from build123d import *

# Parameters (mm, degrees)
F0_W     = 16.8741471134
F0_H     = 2.6543606073
F0_W_2   = 2.2751651704
F0_H_2   = 12.3238116503
F0_W_3   = 16.8741438538
F0_H_3   = 3.0335541815
F0_W_4   = 2.6543606073
F0_H_4   = 3.9815418422
F0_H_5   = 11.5654245019
F0_W_5   = 11.7550231516
F0_W_6   = 7.0150978863
F0_H_6   = 1.8959715962
F0_W_7   = 2.2786548152
F0_H_7   = 3.3179512247
F0_H_8   = 7.4890879914
F0_W_8   = 11.5619385824
F0_W_9   = 2.8439611197
F0_H_9   = 7.7734831721
F0_H_10  = 2.9387557879
F0_H_11  = 8.0578802153
F0_W_10  = 11.3758221269
F1_DEPTH = 7.62
F2_DEPTH = 8.382
F4_DEPTH = 25.4


with BuildPart() as f1:
    # F0 (on Front) → F1 (new body)
    with BuildSketch(Plane.XZ):
        Polygon((-41.2373803556, 39.1518138349), (-41.2373803556, 41.4269790053), (-46.7357002199, 41.4269790053), (-52.4236150086, 39.5310074091), (-54.8883751035, 35.1702719927), (-54.8883751035, 26.8279965967), (-54.8883751035, 18.2961262763), (-50.5276434124, 15.2625711635), (-46.1669079959, 15.2625711635), (-41.9957712293, 15.2625711635), (-35.9286628664, 15.2625711635), (-30.6199416518, 15.0729743764), (-35.7390642166, 18.2961262763), (-41.2373803556, 18.2961262763), (-49.5796576142, 18.2961262763), (-52.4236150086, 20.3816946596), (-52.4236150086, 25.8800126612), (-52.4236150086, 34.0326912701), (-50.7172383368, 36.8766486645), (-45.2189221978, 39.1518138349), align=None)
        Polygon((-35.7390642166, 34.7910784185), (-35.7390642166, 18.2961262763), (-30.6199416518, 15.0729743764), (-20.9504868835, 15.0729743764), (-17.5377372652, 18.2961262763), (-15.4521688819, 21.7088758945), (-15.4521688819, 32.5159132481), (-15.4521688819, 38.2038280368), (-17.5377372652, 41.6165776551), (-23.415248841, 41.6165776551), (-27.3967888206, 41.4269790053), (-31.9471210241, 41.4269790053), (-35.1702719927, 38.3934266865), align=None)
        Polygon((-17.5377372652, 18.2961262763), (-20.9504868835, 15.0729743764), (-10.1434476674, 15.0729743764), (-10.1434476674, 17.5377372652), align=None)
        Polygon((-10.1434476674, 17.5377372652), (-10.1434476674, 15.0729743764), (-7.6786852442, 14.883376658), (-7.6786852442, 17.5377372652), (-7.6786852442, 36.3078564405), (-10.1434476674, 36.3078564405), align=None)
        with Locations((0.7583883125, 16.2105569616)):
            Rectangle(F0_W, F0_H)
        Polygon((-10.1434476674, 40.2893982828), (-10.1434476674, 36.3078564405), (-7.6786852442, 36.3078564405), (2.3699654266, 36.3078564405), (2.3699654266, 40.2893982828), (-7.8682824969, 40.2893982828), align=None)
        Polygon((9.1954618692, 17.5377372652), (9.1954618692, 14.883376658), (11.8498224765, 14.6937798709), (11.8498224765, 17.7273340523), (11.8498224765, 36.6870500147), (9.1954618692, 36.6870500147), align=None)
        with Locations((-9.0058650821, 46.4513041079)):
            Rectangle(F0_W_2, F0_H_2)
        with Locations((20.2868944034, 16.2105569616)):
            Rectangle(F0_W_3, F0_H_3)
        Polygon((-10.1434476674, 56.0259595513), (-10.1434476674, 52.613209933), (-7.8682824969, 52.613209933), (6.9202957675, 52.613209933), (6.9202957675, 56.0259595513), align=None)
        with Locations((10.5226421729, 38.6778209358)):
            Rectangle(F0_W_4, F0_H_4)
        Polygon((28.7239663303, 17.7273340523), (28.7239663303, 14.6937798709), (42.5645597279, 14.6937798709), (42.5645597279, 16.5897514671), (42.5645597279, 18.1065294892), (31.0026211455, 17.789763132), align=None)
        with Locations((10.5226421729, 46.4513041079)):
            Rectangle(F0_W_4, F0_H_5)
        with Locations((17.7273340523, 38.6778209358)):
            Rectangle(F0_W_5, F0_H_4)
        Polygon((28.7239663303, 25.5008172244), (28.7239663303, 17.7273340523), (31.0026211455, 17.789763132), (31.0026211455, 25.5008172244), align=None)
        with Locations((46.0721086711, 15.641765669)):
            Rectangle(F0_W_6, F0_H_6)
        Polygon((9.1954618692, 56.0259595513), (9.1954618692, 52.2340163589), (11.8498224765, 52.2340163589), (26.2592080981, 52.2340163589), (26.2592080981, 56.0259595513), align=None)
        with Locations((29.8632937379, 27.1597928368)):
            Rectangle(F0_W_7, F0_H_7)
        Polygon((49.5796576142, 16.5897514671), (49.5796576142, 14.6937798709), (63.6098459363, 14.6937798709), (63.6098459363, 18.1065294892), (52.4236187339, 18.1065294892), (49.5796576142, 18.1065294892), align=None)
        with Locations((29.8632937379, 32.5633124448)):
            Rectangle(F0_W_7, F0_H_8)
        with Locations((36.7835904367, 27.1597928368)):
            Rectangle(F0_W_8, F0_H_7)
        Polygon((28.7239663303, 39.9102028459), (28.7239663303, 36.3078564405), (31.0026211455, 36.3078564405), (42.5645597279, 36.3078564405), (42.5645597279, 39.9102028459), align=None)
        with Locations((51.0016381741, 21.9932710752)):
            Rectangle(F0_W_9, F0_H_9)
        with Locations((51.0016381741, 27.3493905552)):
            Rectangle(F0_W_9, F0_H_10)
        with Locations((51.0016381741, 32.8477085568)):
            Rectangle(F0_W_9, F0_H_11)
        with Locations((58.1115297973, 27.3493905552)):
            Rectangle(F0_W_10, F0_H_10)
        Polygon((49.5796576142, 39.9102047086), (49.5796576142, 36.8766486645), (52.4236187339, 36.8766486645), (63.9890432358, 36.8766486645), (63.9890432358, 39.9102047086), align=None)
    extrude(amount=F1_DEPTH)

    # F0 (on Front) → F2 (join)
    with BuildSketch(Plane.XZ):
        Polygon((-41.2373803556, 39.1518138349), (-41.2373803556, 41.4269790053), (-46.7357002199, 41.4269790053), (-52.4236150086, 39.5310074091), (-54.8883751035, 35.1702719927), (-54.8883751035, 26.8279965967), (-54.8883751035, 18.2961262763), (-50.5276434124, 15.2625711635), (-46.1669079959, 15.2625711635), (-41.9957712293, 15.2625711635), (-35.9286628664, 15.2625711635), (-30.6199416518, 15.0729743764), (-35.7390642166, 18.2961262763), (-41.2373803556, 18.2961262763), (-49.5796576142, 18.2961262763), (-52.4236150086, 20.3816946596), (-52.4236150086, 25.8800126612), (-52.4236150086, 34.0326912701), (-50.7172383368, 36.8766486645), (-45.2189221978, 39.1518138349), align=None)
        Polygon((-35.7390642166, 34.7910784185), (-35.7390642166, 18.2961262763), (-30.6199416518, 15.0729743764), (-20.9504868835, 15.0729743764), (-17.5377372652, 18.2961262763), (-15.4521688819, 21.7088758945), (-15.4521688819, 32.5159132481), (-15.4521688819, 38.2038280368), (-17.5377372652, 41.6165776551), (-23.415248841, 41.6165776551), (-27.3967888206, 41.4269790053), (-31.9471210241, 41.4269790053), (-35.1702719927, 38.3934266865), align=None)
        Polygon((-17.5377372652, 18.2961262763), (-20.9504868835, 15.0729743764), (-10.1434476674, 15.0729743764), (-10.1434476674, 17.5377372652), align=None)
        Polygon((-10.1434476674, 17.5377372652), (-10.1434476674, 15.0729743764), (-7.6786852442, 14.883376658), (-7.6786852442, 17.5377372652), (-7.6786852442, 36.3078564405), (-10.1434476674, 36.3078564405), align=None)
        with Locations((0.7583883125, 16.2105569616)):
            Rectangle(F0_W, F0_H)
        Polygon((-10.1434476674, 40.2893982828), (-10.1434476674, 36.3078564405), (-7.6786852442, 36.3078564405), (2.3699654266, 36.3078564405), (2.3699654266, 40.2893982828), (-7.8682824969, 40.2893982828), align=None)
        Polygon((9.1954618692, 17.5377372652), (9.1954618692, 14.883376658), (11.8498224765, 14.6937798709), (11.8498224765, 17.7273340523), (11.8498224765, 36.6870500147), (9.1954618692, 36.6870500147), align=None)
        with Locations((-9.0058650821, 46.4513041079)):
            Rectangle(F0_W_2, F0_H_2)
        with Locations((20.2868944034, 16.2105569616)):
            Rectangle(F0_W_3, F0_H_3)
        Polygon((-10.1434476674, 56.0259595513), (-10.1434476674, 52.613209933), (-7.8682824969, 52.613209933), (6.9202957675, 52.613209933), (6.9202957675, 56.0259595513), align=None)
        with Locations((10.5226421729, 38.6778209358)):
            Rectangle(F0_W_4, F0_H_4)
        Polygon((28.7239663303, 17.7273340523), (28.7239663303, 14.6937798709), (42.5645597279, 14.6937798709), (42.5645597279, 16.5897514671), (42.5645597279, 18.1065294892), (31.0026211455, 17.789763132), align=None)
        with Locations((10.5226421729, 46.4513041079)):
            Rectangle(F0_W_4, F0_H_5)
        with Locations((17.7273340523, 38.6778209358)):
            Rectangle(F0_W_5, F0_H_4)
        Polygon((28.7239663303, 25.5008172244), (28.7239663303, 17.7273340523), (31.0026211455, 17.789763132), (31.0026211455, 25.5008172244), align=None)
        with Locations((46.0721086711, 15.641765669)):
            Rectangle(F0_W_6, F0_H_6)
        Polygon((9.1954618692, 56.0259595513), (9.1954618692, 52.2340163589), (11.8498224765, 52.2340163589), (26.2592080981, 52.2340163589), (26.2592080981, 56.0259595513), align=None)
        with Locations((29.8632937379, 27.1597928368)):
            Rectangle(F0_W_7, F0_H_7)
        Polygon((49.5796576142, 16.5897514671), (49.5796576142, 14.6937798709), (63.6098459363, 14.6937798709), (63.6098459363, 18.1065294892), (52.4236187339, 18.1065294892), (49.5796576142, 18.1065294892), align=None)
        with Locations((29.8632937379, 32.5633124448)):
            Rectangle(F0_W_7, F0_H_8)
        with Locations((36.7835904367, 27.1597928368)):
            Rectangle(F0_W_8, F0_H_7)
        Polygon((28.7239663303, 39.9102028459), (28.7239663303, 36.3078564405), (31.0026211455, 36.3078564405), (42.5645597279, 36.3078564405), (42.5645597279, 39.9102028459), align=None)
        with Locations((51.0016381741, 21.9932710752)):
            Rectangle(F0_W_9, F0_H_9)
        with Locations((51.0016381741, 27.3493905552)):
            Rectangle(F0_W_9, F0_H_10)
        with Locations((51.0016381741, 32.8477085568)):
            Rectangle(F0_W_9, F0_H_11)
        with Locations((58.1115297973, 27.3493905552)):
            Rectangle(F0_W_10, F0_H_10)
        Polygon((49.5796576142, 39.9102047086), (49.5796576142, 36.8766486645), (52.4236187339, 36.8766486645), (63.9890432358, 36.8766486645), (63.9890432358, 39.9102047086), align=None)
    extrude(amount=F2_DEPTH)

    # F3 (on face) → F4 (cut)
    with BuildSketch(Plane.XZ.offset(8.382)):
        Polygon((-19.0104637295, 39.5915135741), (-31.1858598143, 39.2533093691), (-33.5532985628, 36.885868758), (-33.5532985628, 32.8274033964), (-33.5532985628, 22.4557705224), (-32.4259474874, 20.5392725766), (-30.6221842766, 19.2991867661), (-20.8142269403, 19.2991867661), (-18.5595247895, 20.6520091742), (-17.3194371164, 22.4557705224), (-17.3194371164, 32.8274033964), (-17.3194371164, 37.6750156283), align=None)
    extrude(amount=-F4_DEPTH, mode=Mode.SUBTRACT)


solid = f1.part
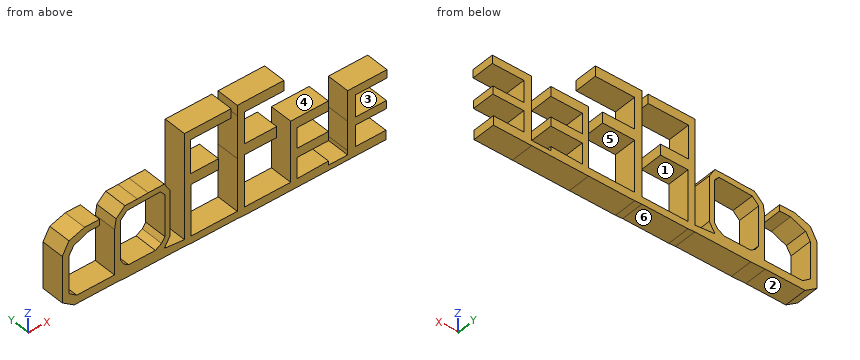
CAD build for the part. Positions are in the model's coordinates, mm. Face numbers are marked on the shaded views. A direction names the side the tool comes from. Round coordinates to 2 decimals unless told otherwise and drop trailing zeros. Order: outer loops, then holes, each group sorted by start corner. A loop starts at its lowest first (then second) coordinate and runs counter-clockwise, first axis right, second up. Notation, with made-up numbers: (45.25, 55) - (95.25, 55) arc R18 ccw to (95.25, 64) - close; hole circle Ø10 at (66.5, 87.25). An arc over 180 degrees is marked (long way). Return JSON: item names as keys, results as strings.
(1) Cut at D-D (x = -22). Give the cut face in (y, z).
Answer key:
{"outline": "(-8.38, 15.07) - (0, 15.07) - (0, 19.3) - (-8.38, 19.3) - close; (-8.38, 39.51) - (0, 39.51) - (0, 41.62) - (-8.38, 41.62) - close"}
(2) Cut at A-A (z = 47). Give the cut face in (x, y), then the cut area to 3 significant figures.
Answer key:
{"outline": "(-10.14, -8.38) - (-7.87, -8.38) - (-7.87, 0) - (-10.14, 0) - close; (9.2, -8.38) - (11.85, -8.38) - (11.85, 0) - (9.2, 0) - close", "area": "41.3 mm^2"}
(3) Tool access for the marked faces 1, 2 and 3: list every direction of +Z, -Z, +X, -X, +Y, -Y with a clear straight run to the whole face (end or side of a thin tool).
Answer key:
{"face 1": "+Y, -Y", "face 2": "-Z, -X, +Y, -Y", "face 3": "+X, +Y, -Y"}
(4) Cut at B-B (x = 35). Give the cut face in (y, z), then the cut area to 3 significant figures.
Answer key:
{"outline": "(-8.38, 14.69) - (0, 14.69) - (0, 17.9) - (-8.38, 17.9) - close; (-8.38, 25.5) - (0, 25.5) - (0, 28.82) - (-8.38, 28.82) - close; (-8.38, 36.31) - (0, 36.31) - (0, 39.91) - (-8.38, 39.91) - close", "area": "84.9 mm^2"}
(5) Pin check, flat tips, straight feed: pin 1 Ø4 at (y, z) = (-3.5, 21.5) entering from +X; pin 2 Ø4 at (x, y) = (-9.5, -5.5) entering from -Z; pin 3 Ø4 at (y, z) = (-4, 16) entering from +X; pin 4 Ø6 at (x, z) = (4.5, 44.5) entering from +Y. Stop position of each tip, or through.
Answer key:
{"pin 1": "stops at x = 52.42", "pin 2": "stops at z = 14.88", "pin 3": "stops at x = 63.61", "pin 4": "passes through"}
(6) Wall check: probe 1 along Z at (x, y) = (-6.5, -2.75); probe 2 along Z at (x, y) = (52.5, -0.75); probe 3 along X at (y, z) = (-6.5, 53). Give the ranges that are in metal, low to high. Write a range as from..to.
Answer key:
{"probe 1": "z = 14.88..17.54, 36.31..40.29, 52.61..56.03", "probe 2": "z = 14.69..18.11, 25.88..28.82, 36.88..39.91", "probe 3": "x = -10.14..6.92, 9.2..26.26"}
(7) Cut at C-C (z = 32.5). Give the cut face in (x, y).
Answer key:
{"outline": "(-54.89, -8.38) - (-52.42, -8.38) - (-52.42, 0) - (-54.89, 0) - close; (-35.74, -8.38) - (-33.55, -8.38) - (-33.55, 0) - (-35.74, 0) - close; (-17.32, -8.38) - (-15.45, -8.38) - (-15.45, 0) - (-17.32, 0) - close; (-10.14, -8.38) - (-7.68, -8.38) - (-7.68, 0) - (-10.14, 0) - close; (9.2, -8.38) - (11.85, -8.38) - (11.85, 0) - (9.2, 0) - close; (28.72, -8.38) - (31, -8.38) - (31, 0) - (28.72, 0) - close; (49.58, -8.38) - (52.42, -8.38) - (52.42, 0) - (49.58, 0) - close"}
(8) Pull direction Z, two halves, no side cores. Call the marked faces 4, 5 and 6: +Z half, -Z half, draft (parallel to the pull), parting line (faces both ways), or undercut.
Answer key:
{"face 4": "+Z half", "face 5": "undercut", "face 6": "-Z half"}
